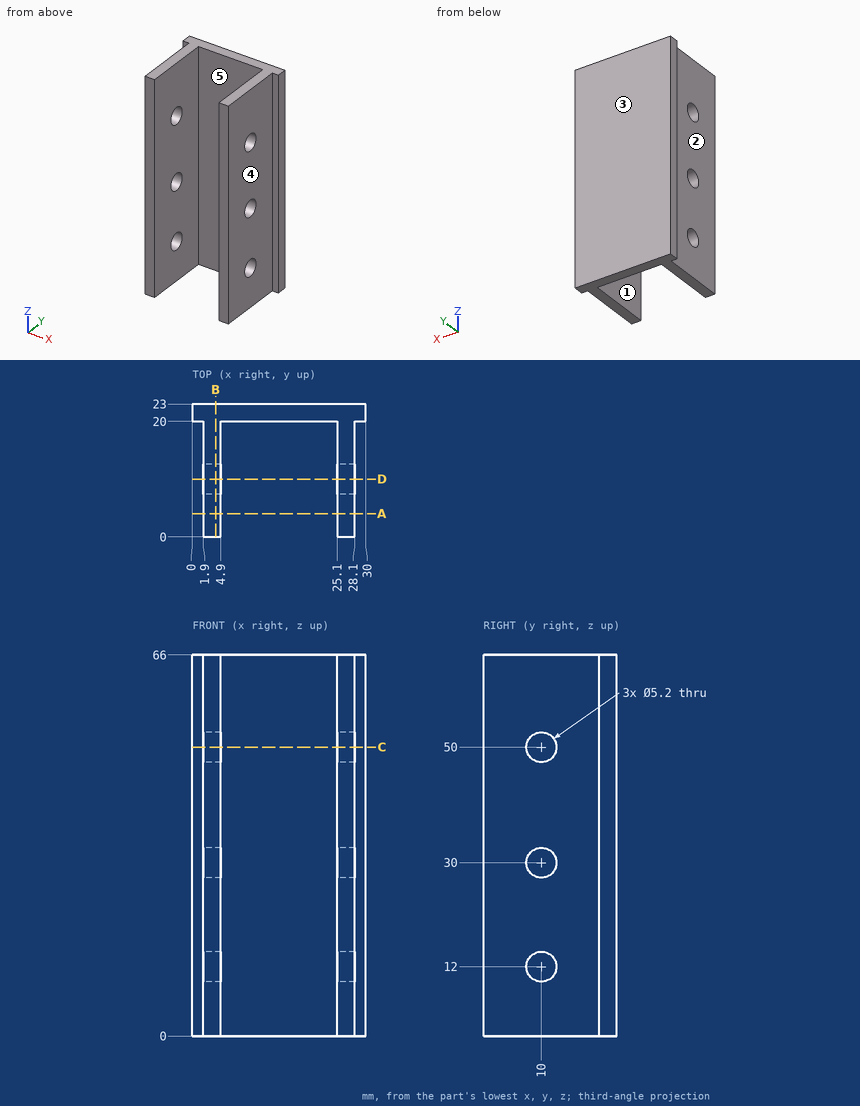
Design review of the part shown in the three views and the two pictorial views. Dimensions are in mm from the part's minimum x, y and z. A direction names the side the tool comes from. Coordinates: 2 decimals unless noted, no trailing zeros. Write each loop counter-clockwise with the first axis right and the second up, starting at its lowest first coordinate (ties: lowest second). Pieces come first, ordered by that corner, then holes.
1) Clearance check with flat-ended pins moving along their axes: pin 1 Ø7 at (y, z) = (10, 30) entering from -X; pin 2 Ø10 at (y, z) = (7.5, 27) entering from +X; pin 3 Ø4.5 at (y, z) = (10, 12) entering from +X; pin 4 Ø0.6 at (x, z) = (1, 25) entering from -Y. State where each tip first meets the part, or that it passes through.
2) We need section A-A on y = 4. State the section outline as (x, z) points, then the cut area to 3 significant figures.
3) We need section D-D on y = 10. Count the separate pieces of the cut face and the enclosed holes in it, then the cut area to 3 significant figures.
4) To check wall thickness, follow probe 1 along X at (y, z) = (8, 41); probe 2 along Y at (x, z) = (26.85, 12); probe 3 along Z at (x, y) = (25.25, 9.5). State the ranges of each line that lie inside material, in increasing order.
5) The part is to be moulded in two halves that separate along X. For the marked faces 1, 2 and 3, say which applies: pulls with the +X half, pulls with the -X half, needs draft (parallel to the pull), parting line crosses it, or undercut.
6) We need section B-B on x = 4. State the section outline as (y, z) points, then the cut area to 3 significant figures.
7) Machinability: for the marked faces 4 and 5, which of the approach directions +Z, -Z, +X, -X, +Y, -Y give a long, thin tool a straight path to every point of the face, cutting with its end or side? Answer none if there is none.
8) We need section C-C on z = 50. State the section outline as (x, y) points, then the cut area to 3 significant figures.
Answer list:
1. pin 1: stops at x = 1.9
1. pin 2: stops at x = 28.1
1. pin 3: passes through
1. pin 4: stops at y = 20
2. outline: (1.9, 0) - (4.9, 0) - (4.9, 66) - (1.9, 66) - close; (25.1, 0) - (28.1, 0) - (28.1, 66) - (25.1, 66) - close
2. area: 396 mm2
3. separate pieces: 8
3. enclosed holes: 0
3. area: 302 mm2
4. probe 1: x = 1.9 to 4.9, 25.1 to 28.1
4. probe 2: y = 0 to 7.4, 12.6 to 23
4. probe 3: z = 0 to 9.45, 14.55 to 27.45, 32.55 to 47.45, 52.55 to 66
5. face 1: undercut
5. face 2: pulls with the -X half
5. face 3: needs draft
6. outline: (0, 0) - (23, 0) - (23, 66) - (0, 66) - close; hole circle Ø5.2 at (10, 12); hole circle Ø5.2 at (10, 30); hole circle Ø5.2 at (10, 50)
6. area: 1,450 mm2
7. face 4: +Z, -Z, +X, -Y
7. face 5: +Z, -Z, -Y
8. outline: (0, 20) - (1.9, 20) - (1.9, 12.6) - (4.9, 12.6) - (4.9, 20) - (25.1, 20) - (25.1, 12.6) - (28.1, 12.6) - (28.1, 20) - (30, 20) - (30, 23) - (0, 23) - close; (1.9, 0) - (4.9, 0) - (4.9, 7.4) - (1.9, 7.4) - close; (25.1, 0) - (28.1, 0) - (28.1, 7.4) - (25.1, 7.4) - close
8. area: 179 mm2
